Job drawing, mm, ordinate dimensions from the low corner. One solid piece. A direction names the side the tool comes from. Round coordinates to 2 decimals unless told otherwise and drop trailing zeros. Order: outer loops, then holes, each group sorted by start corner. A loop starts at its lowest first (then second) coordinate and runs counter-clockwise, first axis right, second up. Notation, with made-up numbers: (11, 43) -> (15, 43) arc R9 cw to (15, 50) -> close; hole circle Ø1 at (83, 71.25). An arc over 180 degrees is marked (long way). Return JSON: item names as keys, results as strings. Group by question number.
Q1. Cut at A-A (x = 10). Write the cut outline in (y, z).
Q2. Which spindle directions (+Z, -Z, +X, -X, +Y, -Y) get a long thin tool onto all of the face, cutting with end or side? Do the marked faces 4, 5 and 6. Say none if no direction does.
Q3. Probe line 1 along Y through (x, z) = (10, 4.25); line 2 along Y through (x, z) = (26, 3.8); line 3 along X through (y, z) = (26, 2.25). List the from-to ranges inside material, lowest first.
Q4. Flat gauge pins, fed straight in: pin 1 (3 mm diameter, centred on x = 10, y = 26, fed in from -Z); pin 2 (1.8 mm diameter, centred on x = 27, y = 11, fed in from +Z); pin 3 (3 mm diameter, centred on x = 16, y = 10.5, fed in from -Z); pin 4 (5.5 mm diameter, centred on x = 24.5, z = 3, fed in from +Y). Where does each tip first touch, or does it go through?
Q5. Mould opens along Y. For the marked faces 1, 2 and 3 say: +Y half, -Y half, draft (parallel to the pull), parting line (faces both ways), or undercut.
Q6. Cut at C-C (x = 26). Write the cut outline in (y, z).
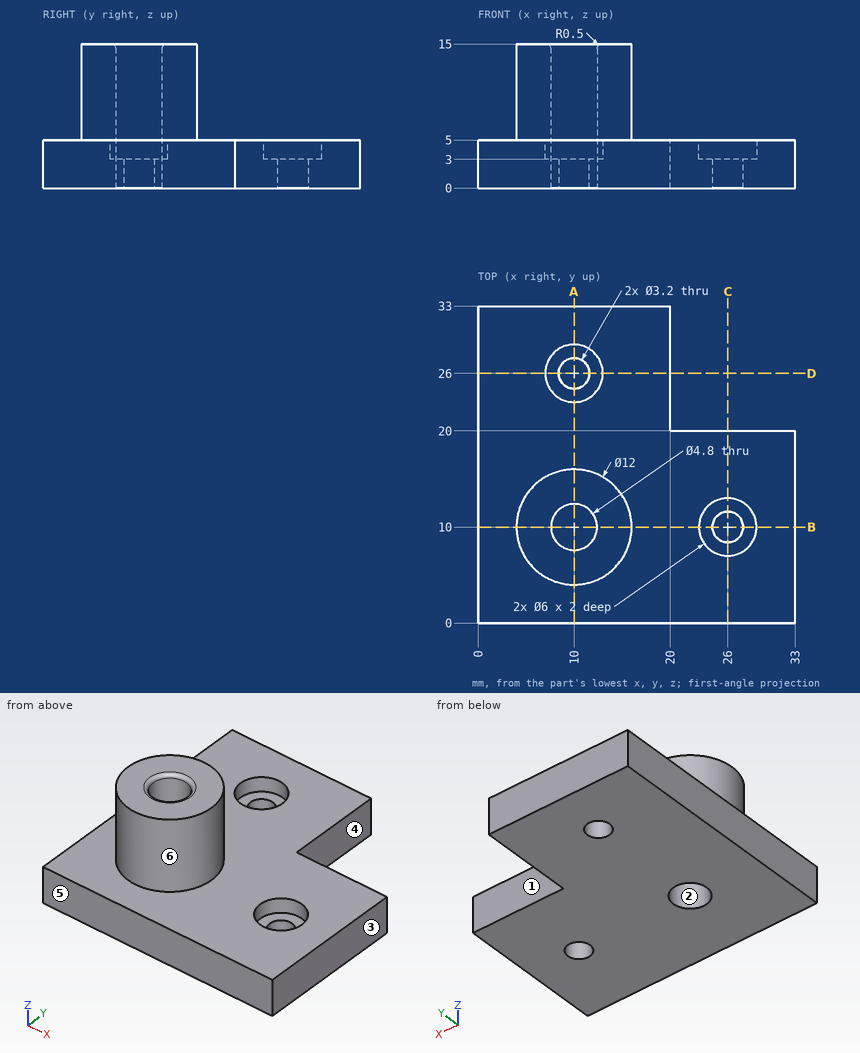
Solution:
{
 "1": {"outline": "(0, 0) -> (7.6, 0) -> (7.6, 14.5) arc R0.5 ccw to (7.1, 15) -> (4, 15) -> (4, 5) -> (0, 5) -> close; (12.4, 0) -> (24.4, 0) -> (24.4, 3) -> (23, 3) -> (23, 5) -> (16, 5) -> (16, 15) -> (12.9, 15) arc R0.5 ccw to (12.4, 14.5) -> close; (27.6, 0) -> (33, 0) -> (33, 5) -> (29, 5) -> (29, 3) -> (27.6, 3) -> close"},
 "2": {"face 4": "+Z, -Z, +X, +Y", "face 5": "+Z, -Z, +X, -X, -Y", "face 6": "+Z"},
 "3": {"line 1": "y = 0 to 7.6, 12.4 to 23, 29 to 33", "line 2": "y = 0 to 7, 13 to 20", "line 3": "x = 0 to 8.4, 11.6 to 20"},
 "4": {"pin 1": "passes through", "pin 2": "stops at z = 3", "pin 3": "stops at z = 0", "pin 4": "stops at y = 20"},
 "5": {"face 1": "+Y half", "face 2": "undercut", "face 3": "draft"},
 "6": {"outline": "(0, 0) -> (8.4, 0) -> (8.4, 3) -> (7, 3) -> (7, 5) -> (0, 5) -> close; (11.6, 0) -> (20, 0) -> (20, 5) -> (13, 5) -> (13, 3) -> (11.6, 3) -> close"}
}
